Autodesk Inventor part; units mm, degrees
ref_plane "YZ Plane" through (0, 0, 0) normal (1, 0, 0) x (0, 1, 0)
ref_plane "XZ Plane" through (0, 0, 0) normal (0, 1, 0) x (-1, 0, 0)
ref_plane "XY Plane" through (0, 0, 0) normal (0, 0, 1) x (1, 0, 0)
sketch "Sketch1" plane through (0, 0, 0) normal (0, 1, 0) x (-1, 0, 0)
  line L0 (12.5, 15) -> (-12.5, 15)
  line L1 (-12.5, 15) -> (-12.5, -15)
  line L2 (-12.5, -15) -> (12.5, -15)
  line L3 (12.5, -15) -> (12.5, 15)
  line L4 (12.5, 15) -> (-12.5, -15) construction
  line L5 (-12.5, 15) -> (12.5, -15) construction
  point P0 (0, 0)
  dimension "d0" = 25
  dimension "d1" = 30
extrude "Extrusion1" add sketch "Sketch1" along normal blind 4
sketch "Sketch2" plane through (0, 4, 0) normal (0, 1, 0) x (1, 0, 0)
  line L0 (-12.5, 15) -> (-12.5, -15) construction
  line L1 (-12.5, -11) -> (12.5, -11) construction
  line L2 (12.5, -15) -> (12.5, 15) construction
  line L3 (-12.5, -15) -> (12.5, -15) construction
  circle A0 centre (0, -4) radius 7
  line L4 (0, -15) -> (0, 15) construction
  line L5 (12.5, 15) -> (-12.5, 15) construction
  point P0 (0, 0)
  point P1 (0, -11)
  dimension "d5" = 14
  dimension "d4" = 4
extrude "Extrusion2" cut sketch "Sketch2" against normal through all
sketch "Sketch3" plane through (0, 0, 0) normal (1, 0, 0) x (0, 1, 0)
  line L0 (4, -3) -> (4, 11) construction
  line L1 (0, -15) -> (0, 15) construction
  line L2 (0, 15) -> (4, 15) construction
  line L3 (4, -15) -> (4, 15) construction
  line L4 (0, -15) -> (4, -15) construction
  line L5 (4, 4) -> (0, 4) construction
  line L6 (2, 4) -> (0.5, 5.258649)
  line L7 (2, 4) -> (2, -15)
  line L8 (0, -15) -> (4, -15)
  line L9 (2, -15) -> (1.618278, -15)
  line L10 (0.5, 15) -> (0.5, 5.258649)
  line L11 (1.618278, -15) -> (0, -15)
  line L12 (0, -15) -> (0, 15)
  line L13 (0, 15) -> (0.5, 15)
  line L14 (0, 15) -> (4, 15)
  line L15 (4, 11) -> (0, 11)
  line L16 (4, -3) -> (0, -3)
  point P0 (0, 0)
  dimension "d6" = 50
  dimension "d7" = 2
  dimension "d8" = 1.5
extrude "Extrusion3" cut sketch "Sketch3" along normal through all both and the other way through all
sketch "Sketch7" plane through (-12.5, 4, 15) normal (0, 0, 1) x (1, 0, 0)
  line L0 (0, -3.5) -> (25, -3.5) construction
  line L1 (25, -3.5) -> (25, 0) construction
  line L2 (0, 0) -> (25, 0) construction
  line L3 (0, -3.5) -> (0, 0) construction
  line L4 (5.5, -2) -> (19.5, -2) construction
  circle A0 centre (12.5, -2) radius 0.875 construction
  line L5 (12.5, -2) -> (14.5, -2) construction
  line L6 (12.5, 0) -> (12.5, -3.5) construction
  line L7 (12.5, -2) -> (10.5, -2) construction
  spline S0 degree 5 poles (10.5, -2) (10.5, -1.67732) (11.1, -1.13952) (13.34, -0.733036) (15.98, -2) (13.34, -3.266964) (11.1, -2.86048) (10.5, -2.32268) (10.5, -2) knots 0 0 0 0 0 0 0.3 0.5 0.7 1 1 1 1 1 1
  line L8 (10.5, -2) -> (10.5, 0)
  line L9 (14.5, -2) -> (14.5, 0)
  line L10 (10.5, 0) -> (14.5, 0)
  point P0 (12.5, -4)
  point P1 (12.5, -2.875)
  dimension "d26" = 1.75
  dimension "d27" = 2
  dimension "d28" = 2
extrude "Extrusion4" cut sketch "Sketch7" against normal blind 10.25
sketch "Sketch4" plane through (0, 0, 0) normal (1, 0, 0) x (0, 1, 0)
  line L0 (2, -15) -> (2, 4)
  line L1 (2, 4) -> (0.5, 5.258649)
  line L2 (0.5, 5.258649) -> (0.5, 15)
  line L3 (0.5, 15) -> (4, 15)
  line L4 (4, -15) -> (4, 15)
  line L5 (2, -15) -> (4, -15)
  line L6 (4, 11) -> (4, -3)
  line L7 (2, 4) -> (2, -15)
  line L8 (4, 4) -> (0, 4)
  line L9 (4, -15) -> (4, 15)
  line L10 (2, 4.5) -> (2, 3.5)
  line L11 (2.965926, 4.758819) -> (1.034074, 4.241181)
  line L12 (1.034074, 4.241181) -> (6.725631, -17)
  line L13 (6.725631, -17) -> (8.657483, -16.482362)
  line L14 (8.657483, -16.482362) -> (3.169251, 4)
  line L15 (3.169251, 4) -> (1.098698, 4)
  point P0 (0, 0)
  point P1 (2, 4)
  dimension "d13" = 0.5
  dimension "d18" = 15
  dimension "d19" = 2
  dimension "d20" = 2
revolve "Revolution2" cut sketch "Sketch4" angle 360 about axis through (0, 4, 4) along (0, -1, 0) contours L0 L12 L8 | L0 L8 L14 L4 L12 | L4 L14 L13 L12
properties part number "wide_access_platform_v01_ok"
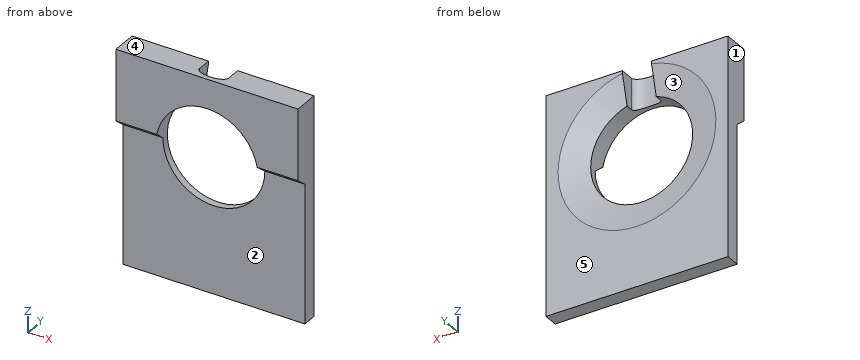
Here's how the part is built. I have some questions about the finished solid (model axes, mm). Face numbers are marked on the shaded views. A direction names the side the tool comes from. Give positions to 0.01 mm unless a question says otherwise; leave off trailing zeros. Order: outer loops, then holes, each group sorted by start corner. A loop starts at its lowest first (then second) coordinate and runs counter-clockwise, first axis right, second up. Notation, with made-up numbers: (19, -27.75) - (24, -27.75) arc R22 ccw to (24, -4.75) - close; hole circle Ø3 at (-12.5, 9.25). An arc over 180 degrees is marked (long way). Answer as a JSON object with one key per item and string values. Group by question number.
Item 1: Please list where these lines run through material, in increasing order: probe 1 along Y at (x, z) = (-11, -10.5); probe 2 along Z at (x, y) = (0, 2.45); probe 3 along X at (y, z) = (2.9, 6).
Item 2: Which directions (+Z, -Z, +X, -X, +Y, -Y) give clear straight access to the entire face, cutting with the end or side of a thin tool? Please do the marked faces 1 and 2.
Item 3: For P1, Ø1.5, axis at x = 9, y = 1, coming from the -Z side; P2, Ø8, axis at x = 8.5, z = -1.5, coming from the -Y side; P3, Ø3, axis at x = 4, z = 1.5, coming from the +Y side, each with a flat end and sliding along its axis, tell me the tip position at first contact or that it passes through.
Item 4: If we section it at A-A on y = 3.6: Please give me the cut outline in (x, z).
Item 5: If we mould it in two halves opening along Z, with no side actions, what happens to the marked faces 3, 4 and 5? For each: pulls with the +Z half, pulls with the -Z half, needs draft (parallel to the pull), parting line crosses it, or undercut.
Result set:
{
 "1": {"probe 1": "2 to 4", "probe 2": "-15 to -3", "probe 3": "-12.5 to -6.71, 6.71 to 12.5"},
 "2": {"face 1": "+Z, -Z, -X, +Y, -Y", "face 2": "-Z, +X, -X, -Y"},
 "3": {"P1": "z = 4.21", "P2": "y = 2", "P3": "through"},
 "4": {"outline": "(-12.5, -15) - (12.5, -15) - (12.5, 15) - (2, 15) - (2, 13.12) arc R9.33 cw (long way) to (-2, 13.12) - (-2, 15) - (-12.5, 15) - close"},
 "5": {"face 3": "undercut", "face 4": "pulls with the +Z half", "face 5": "needs draft"}
}
